Here's the drawing with two shaded views (mm, measured from the low corner). I have some questions. A direction names the side the tool comes from. Give positions to 0.01 mm unless a question says otherwise; leave off trailing zeros. Order: outer loops, then holes, each group sorted by start corner. A loop starts at its lowest first (then second) coordinate and runs counter-clockwise, first axis right, second up. Notation, with made-up numbers: M -1.75,-13 L 47.25,-13 A31 ccw 47.25,19 Z; hole C 0,62.5 d4. An arc over 180 degrees is marked long. Use a Markdown table: item, result. Add a question column.
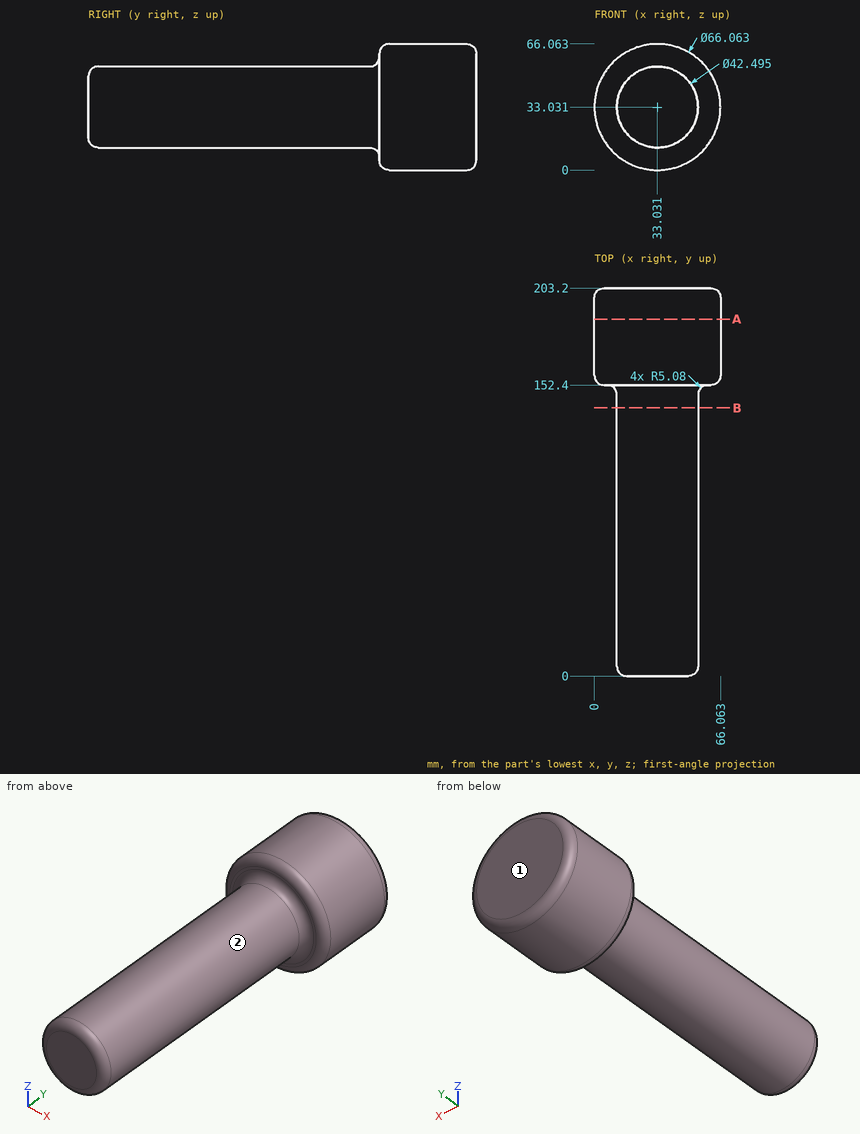
1. I need wall thicknesses on L1, parallel to Y at x = 26.5, z = 58.5; L2, parallel to Z at x = 33, y = 122.5 (1 decimal); L3, parallel to Z at x = 42, y = 129.5 (1 decimal). Which ranges of each line are inside material? Lowest first, please. Write a range as [from, to].
2. On a 3-axis mill with a long thin cutter (end or side, diameter ignored), from which of +Z, -Z, +X, -X, +Y, -Y can I reach the whole of each face in a straight line? I mean the marked faces 1 and 2. Say none if no direction works.
3. If we section it at B-B, the plane y = 140.5: List the corners of the cut face in (x, z) for me (1 decimal), then the cut area to 3 significant figures.
4. If we section it at A-A, the plane y = 187: List the corners of the cut face in (x, z) for me.
5. Will these pins go through, and if not, where does the flat tip stop? pin 1 (5 mm diameter, centred on x = 24.5, y = 165, fed in from +Z); pin 2 (4 mm diameter, centred on y = 32, z = 53.5, fed in from -X) (1 decimal); pin 3 (5 mm diameter, centred on x = 39, y = 63.5, fed in from -Z).
Geometry results:
| question | item | result |
|---|---|---|
| 1 | L1 | y = [152.4, 203.2] |
| 1 | L2 | z = [11.8, 54.3] |
| 1 | L3 | z = [13.8, 52.3] |
| 2 | face 1 | +Z, -Z, +X, -X, +Y |
| 2 | face 2 | -Y |
| 3 | outline | C 33,33 d42.5 |
| 3 | area | 1,420 mm^2 |
| 4 | outline | C 33.03,33.03 d66.06 |
| 5 | pin 1 | stops at z = 65.51 |
| 5 | pin 2 | stops at x = 22.5 |
| 5 | pin 3 | stops at z = 12.07 |
